The figure shows three views and two pictorial views of one solid part (mm, origin at its lowest corner). Answer the questions. A direction names the side the tool comes from. Coordinates: 2 decimals unless noted, no trailing zeros. Order: outer loops, then holes, each group sorted by start corner. A loop starts at its lowest first (then second) coordinate and runs counter-clockwise, first axis right, second up. Notation, with made-up numbers: (1.25, 24) - (19.25, 24) arc R20 ccw to (19.25, 43) - close; hole circle Ø11 at (43, -22). An arc over 180 degrees is marked (long way). Use one line per item in the form item = value.
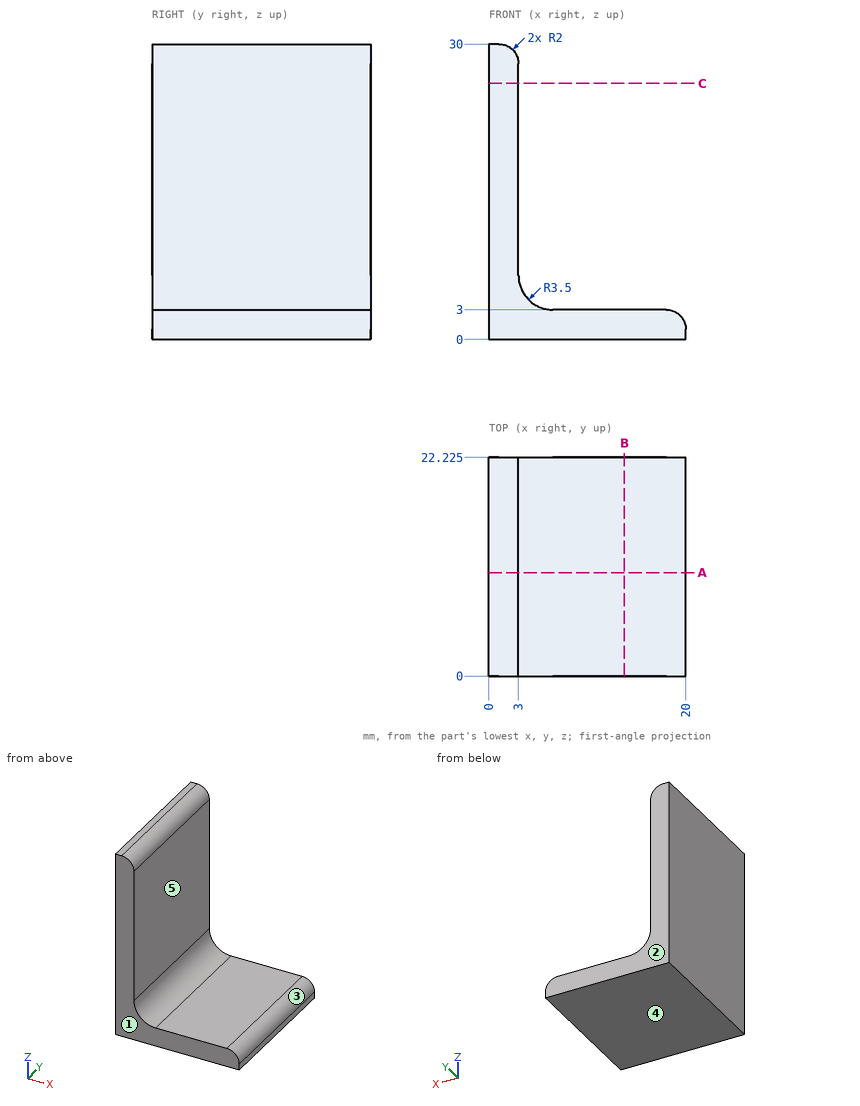
(1) Which of the six approach directions +Z, -Z, +X, -X, +Y, -Y give full straight-line access (tool end or side, diameter ignored) to the marked faces 4 and 5?
Answer list:
face_4 = -Z, +X, -X, +Y, -Y
face_5 = +Z, +X, +Y, -Y
(2) Section A-A, the plane y = 10.5 is taken. Write down the section's boundary in (x, z).
Answer list:
outline = (0, 0) - (20, 0) - (20, 1) arc R2 ccw to (18, 3) - (6.5, 3) arc R3.5 cw to (3, 6.5) - (3, 28) arc R2 ccw to (1, 30) - (0, 30) - close
(3) Straight lines are drawn through the part: L1, parallel to X at y = 18.75, z = 8; L2, parallel to X at y = 11.5, z = 2.75. For each, find the intervals that lie inside material, in ascending order.
Answer list:
L1 = 0 to 3
L2 = 0 to 18.97
(4) Section C-C, the plane z = 26 is taken. Write down the section's boundary in (x, y) (3 decimals), then the cut area to 3 significant figures.
Answer list:
outline = (0, 0) - (3, 0) - (3, 22.225) - (0, 22.225) - close
area = 66.7 mm2
(5) Given pin 1 Ø1.5 at (x, y) = (13, 11) entering from +Z; pin 2 Ø10 at (x, y) = (10, 4.5) entering from +Z, each flat-ended and moving along its own axis, determine where each tip first touches the part or whether it passes through.
Answer list:
pin_1 = 3
pin_2 = 3.34
(6) Section B-B, the plane x = 13.75 is taken. Write down the section's boundary in (y, z) (3 decimals), then the cut area to 3 significant figures.
Answer list:
outline = (0, 0) - (22.225, 0) - (22.225, 3) - (0, 3) - close
area = 66.7 mm2
(7) The mould has two halves that part along Y. Classify the marked faces 1, 2 and 3: +Y half, -Y half, draft (parallel to the pull), parting line (faces both ways), or undercut.
Answer list:
face_1 = -Y half
face_2 = +Y half
face_3 = draft
